```python
from build123d import *

# Parameters (mm, degrees)
BOSS_EXTRUDE1_DEPTH     = 3.7338
BOSS_EXTRUDE2_DEPTH     = 3.7338
CUT_EXTRUDE1_DEPTH      = 197.398400929
FILLET7_R               = 9.525
FILLET8_R               = 3.175
F_8_32_TAPPED_HOLE2_D   = 4.1656
FILLET3_RADIUS          = 1.8669
FILLET3_LENGTH          = 19.05
FILLET4_RADIUS          = 1.8669
FILLET4_LENGTH          = 19.05
FILLET5_RADIUS          = 1.8669
FILLET5_LENGTH          = 19.05
FILLET6_START           = -20
FILLET6_DEPTH           = 25
F_8_CLEARANCE_HOLE1_D   = 4.4958
CUT_EXTRUDE2_DEPTH      = 196.843388239
CUT_EXTRUDE3_DEPTH      = 196.843388239
SKETCH15_W              = 95.363977372
SKETCH15_H              = 7.9375
CUT_EXTRUDE4_DEPTH      = 196.843388239
SKETCH16_W              = 18.936022628
SKETCH16_H              = 6.35
CUT_EXTRUDE5_DEPTH      = 196.843388239
CUT_EXTRUDE6_DEPTH      = 196.843388239
CUT_EXTRUDE6_DEPTH_BACK = 196.843388239
SKETCH17_W              = 3.175
SKETCH17_H              = 3.175
SKETCH18_W              = 25.4
SKETCH18_H              = 3.175
CUT_EXTRUDE7_DEPTH      = 196.843388239


with BuildPart() as part:
    # Sketch1 → Boss-Extrude1 (new body)
    with BuildSketch(Plane.XY):
        Polygon((0, 0), (9.525, 0), (9.525, -19.05), (20.6375, -19.05), (20.6375, 0), (46.0375, 0), (46.0375, -19.05), (180.975, -19.05), (180.975, 3.175), (-16.893133293, 76.2), align=None)
    extrude(amount=BOSS_EXTRUDE1_DEPTH)

    # Sketch7 → Boss-Extrude2 (add)
    with BuildSketch(Plane.XY.offset(3.7338)):
        Polygon((-161.613635382, -74.129081959), (-0.247657199, 1.117109433), (-16.893133293, 76.2), (-166.605179671, -63.424680687), align=None)
    extrude(amount=-BOSS_EXTRUDE2_DEPTH)

    # Sketch8 → Cut-Extrude1 (cut, through all)
    with BuildSketch(Plane.XY.offset(3.7338)):
        Polygon((2.518832326, 10.642109433), (133.231722564, 10.642109433), (-9.128883742, 63.181561352), align=None)
        Polygon((-18.542737866, 61.637057548), (-138.674453357, -50.400369109), (-7.28718114, 10.86652211), align=None)
    extrude(amount=-CUT_EXTRUDE1_DEPTH, mode=Mode.SUBTRACT)

    # Fillet7
    fillet7_edges = [part.edges().sort_by_distance(p)[0] for p in [
        (-16.893133293, 76.2, 1.8669),
    ]]
    fillet(fillet7_edges, radius=FILLET7_R)

    # Fillet8
    fillet8_edges = [part.edges().sort_by_distance(p)[0] for p in [
        (-9.128883742, 63.181561352, 1.8669),
        (133.231722564, 10.642109433, 1.8669),
        (2.518832326, 10.642109433, 1.8669),
        (-7.28718114, 10.86652211, 1.8669),
        (-138.674453357, -50.400369109, 1.8669),
        (-18.542737866, 61.637057548, 1.8669),
    ]]
    fillet(fillet8_edges, radius=FILLET8_R)

    # #8-32 Tapped Hole2 (through all)
    with Locations(Plane.XY.offset(3.7338)):
        with Locations((15.08125, -11.1125), (58.7375, -11.1125), (168.275, -4.7625)):
            Hole(F_8_32_TAPPED_HOLE2_D / 2)

    # Fillet3: full round fillet: the end face becomes a half cylinder, R = half its width
    fillet3_face = Plane((9.525, -9.525, 1.8669), x_dir=(0, 1, 0), z_dir=(-1, 0, 0))  # on the end face: x along it, z out of the body
    fillet3_slab = fillet3_face.offset(-FILLET3_RADIUS / 2) * Box(FILLET3_LENGTH, 2 * FILLET3_RADIUS, FILLET3_RADIUS, mode=Mode.PRIVATE)  # the body's end, R deep
    fillet3_round = Plane((11.3919, -9.525, 1.8669), x_dir=(-1, 0, 0), z_dir=(0, 1, 0)) * Cylinder(FILLET3_RADIUS, FILLET3_LENGTH, mode=Mode.PRIVATE)  # its axis R under the face
    add(fillet3_slab - fillet3_round, mode=Mode.SUBTRACT)

    # Fillet4: full round fillet: the end face becomes a half cylinder, R = half its width
    fillet4_face = Plane((20.6375, -9.525, 1.8669), x_dir=(0, 1, 0), z_dir=(1, 0, 0))  # on the end face: x along it, z out of the body
    fillet4_slab = fillet4_face.offset(-FILLET4_RADIUS / 2) * Box(FILLET4_LENGTH, 2 * FILLET4_RADIUS, FILLET4_RADIUS, mode=Mode.PRIVATE)  # the body's end, R deep
    fillet4_round = Plane((18.7706, -9.525, 1.8669), x_dir=(1, 0, 0), z_dir=(0, 1, 0)) * Cylinder(FILLET4_RADIUS, FILLET4_LENGTH, mode=Mode.PRIVATE)  # its axis R under the face
    add(fillet4_slab - fillet4_round, mode=Mode.SUBTRACT)

    # Fillet5: full round fillet: the end face becomes a half cylinder, R = half its width
    fillet5_face = Plane((46.0375, -9.525, 1.8669), x_dir=(0, -1, 0), z_dir=(-1, 0, 0))  # on the end face: x along it, z out of the body
    fillet5_slab = fillet5_face.offset(-FILLET5_RADIUS / 2) * Box(FILLET5_LENGTH, 2 * FILLET5_RADIUS, FILLET5_RADIUS, mode=Mode.PRIVATE)  # the body's end, R deep
    fillet5_round = Plane((47.9044, -9.525, 1.8669), x_dir=(-1, 0, 0), z_dir=(0, -1, 0)) * Cylinder(FILLET5_RADIUS, FILLET5_LENGTH, mode=Mode.PRIVATE)  # its axis R under the face
    add(fillet5_slab - fillet5_round, mode=Mode.SUBTRACT)

    # Fillet6: read off the stored shape, not the designer's step
    # Fillet6 outline → Fillet6 (cut)
    with BuildSketch(Plane(origin=(0, 0, 0), x_dir=(1, 0, 0), z_dir=(0, 1, 0)).offset(FILLET6_START)):
        with BuildLine():
            ThreePointArc((179.1081, 0), (180.42819765, -0.54680235), (180.975, -1.8669))
            Line((180.975, -1.8669), (180.975, 0))
            Line((180.975, 0), (179.1081, 0))
        make_face()
        with BuildLine():
            ThreePointArc((180.975, -1.8669), (180.42819765, -3.18699765), (179.1081, -3.7338))
            Line((179.1081, -3.7338), (180.975, -3.7338))
            Line((180.975, -3.7338), (180.975, -1.8669))
        make_face()
    extrude(amount=FILLET6_DEPTH, mode=Mode.SUBTRACT)

    # #8 Clearance Hole1 (through all)
    with Locations(Plane.XY.offset(3.7338)):
        with Locations((-158.829891599, -65.073459713), (-124.299564913, -48.97170394)):
            Hole(F_8_CLEARANCE_HOLE1_D / 2)

    # Sketch12 → Cut-Extrude2 (cut, through all)
    with BuildSketch(Plane.XY.offset(3.7338)):
        Polygon((-0.247657199, 1.117109433), (0, 1.232593882), (0, 0), align=None)
    extrude(amount=-CUT_EXTRUDE2_DEPTH, mode=Mode.SUBTRACT)

    # Sketch14 → Cut-Extrude3 (cut, through all)
    with BuildSketch(Plane.XY.offset(3.7338)):
        with BuildLine():
            Line((71.4375, -6.35), (157.276477372, -6.35))
            ThreePointArc((157.276477372, -6.35), (162.038977372, -11.1125), (157.276477372, -15.875))
            Line((157.276477372, -15.875), (71.4375, -15.875))
            ThreePointArc((71.4375, -15.875), (66.675, -11.1125), (71.4375, -6.35))
        make_face()
    extrude(amount=-CUT_EXTRUDE3_DEPTH, mode=Mode.SUBTRACT)

    # Sketch15 → Cut-Extrude4 (cut, through all)
    with BuildSketch(Plane.XY.offset(3.7338)):
        with Locations((114.356988686, -15.08125)):
            Rectangle(SKETCH15_W, SKETCH15_H)
    extrude(amount=-CUT_EXTRUDE4_DEPTH, mode=Mode.SUBTRACT)

    # Sketch16 → Cut-Extrude5 (cut, through all)
    with BuildSketch(Plane.XY.offset(3.7338)):
        with Locations((171.506988686, -15.875)):
            Rectangle(SKETCH16_W, SKETCH16_H)
    extrude(amount=-CUT_EXTRUDE5_DEPTH, mode=Mode.SUBTRACT)

    # Sketch17 → Cut-Extrude6 (cut, two sides: drawn at the far end of the back side and taken through both)
    with BuildSketch(Plane.XY.offset(3.7338).offset(-CUT_EXTRUDE6_DEPTH_BACK)):
        with Locations((19.05, -17.4625)):
            Rectangle(SKETCH17_W, SKETCH17_H)
    extrude(amount=CUT_EXTRUDE6_DEPTH + CUT_EXTRUDE6_DEPTH_BACK, mode=Mode.SUBTRACT)

    # Sketch18 → Cut-Extrude7 (cut, through all)
    with BuildSketch(Plane.XY.offset(3.7338)):
        Polygon((-3.347186663, 3.175), (-2.005373682, 0.297472776), (0, 1.232593882), (0, 0), (9.525, 0), (9.525, 3.175), align=None)
        Polygon((-116.86007736, -49.756930231), (-115.518264379, -52.634457455), (-2.005373682, 0.297472776), (-3.347186663, 3.175), align=None)
        with Locations((33.3375, 1.5875)):
            Rectangle(SKETCH18_W, SKETCH18_H)
        with BuildLine():
            ThreePointArc((157.276477372, -6.35), (160.644073417, -7.744903955), (162.038977372, -11.1125))
            Line((162.038977372, -11.1125), (162.038977372, 3.175))
            Line((162.038977372, 3.175), (66.675, 3.175))
            Line((66.675, 3.175), (66.675, -11.1125))
            ThreePointArc((66.675, -11.1125), (68.069903955, -7.744903955), (71.4375, -6.35))
            Line((71.4375, -6.35), (157.276477372, -6.35))
        make_face()
    extrude(amount=-CUT_EXTRUDE7_DEPTH, mode=Mode.SUBTRACT)


solid = part.part
```
For this review, take the finished solid that the model builds, in its own axes (mm). A direction names the side the tool comes from. Coordinates: 2 decimals unless noted, no trailing zeros. Loops run counter-clockwise (first coordinate to the right, second up) from the corner with the lowest first, then second, coordinate; pieces in that order, holes last. Notation, with made-up numbers: (33.5, 51) - (68.5, 51) arc R15 cw to (68.5, 57) - close; hole circle Ø5 at (43, 28.5). An arc over 180 degrees is marked (long way). Use one line per item in the form item = value. Start each with the question number.
1) Take a section at D-D (z = 2.8). State how many separate pieces and enclosed holes the cut face has, plus the area to 3 significant figures.
2) Take a section at A-A (x = -50.5). State the section outline as (y, z) points, plus the area to 3 significant figures.
3) Take a section at C-C (x = 103.5). State the section outline as (y, z) points (3 decimals).
4) Draft analysis for pull direction Y (two halves, no side actions). For faces 1 (the face through (-72.6, 11.22, 1.89)), 2 (the face through (-92.876, 5.336, 1.893)), 3 (the face through (-7, 6, 0)), state which applies: released by +Y, released by -Y, zero draft, split by the parting line, or undercut.
5) Take a section at B-B (y = 26). State the section outline as (x, z) points, plus the area to 3 significant figures.
6) For pin 1 (1.1 mm diameter, centred on x = 57.5, z = 1.5, fed in from -Y); pin 2 (2 mm diameter, centred on x = -34, z = 3, fed in from -Y); pin 3 (0.9 mm diameter, centred on x = 19.5, z = 0.5, fed in from -Y) (3 decimals), all flat-tipped, find the tip position at first contact; note any pin that passes through.
7) For faces 4 (the face through (-3.02, 35.63, 1.89)), 5 (the face through (86.139, 38.175, 1.841)), list the 3-axis set-ups (+Z, -Z, +X, -X, +Y, -Y) from which the entire face can be reached by the end or side of a thin tool; tool diameter is ignored.
8) To check wall thickness, follow probe 1 along X at (y, z) = (-8.5, 1.45) (3 decimals); probe 2 along Y at (x, z) = (-29, 3.15); probe 3 along Y at (x, z) = (-88, 0.7). State the ranges of each line that lie inside material, in increasing order. Write a range as from..to.
From the geometry:
q1.separate_pieces = 1
q1.enclosed_holes = 7
q1.area = 7,960 mm2
q2.outline = (-18.81, 0) - (-9.28, 0) - (-9.28, 3.73) - (-18.81, 3.73) - close; (31.83, 0) - (44.86, 0) - (44.86, 3.73) - (31.83, 3.73) - close
q2.area = 84.2 mm2
q3.outline = (3.175, 0) - (10.642, 0) - (10.642, 3.734) - (3.175, 3.734) - close; (21.615, 0) - (31.768, 0) - (31.768, 3.734) - (21.615, 3.734) - close
q4.face_1 = undercut
q4.face_2 = released by +Y
q4.face_3 = zero draft
q5.outline = (-70.72, 0) - (-56.75, 0) - (-56.75, 3.73) - (-70.72, 3.73) - close; (-10.64, 0) - (-0.89, 0) - (-0.89, 3.73) - (-10.64, 3.73) - close; (91.62, 0) - (119.13, 0) - (119.13, 3.73) - (91.62, 3.73) - close
q5.area = 191 mm2
q6.pin_1 = -19.05
q6.pin_2 = -11.58
q6.pin_3 = -15.875
q7.face_4 = +Z, -Z
q7.face_5 = +Z, -Z, +X, +Y
q8.probe_1 = -107.712..-93.747, -48.819..-28.384, 9.572..20.59, 46.085..66.675, 162.039..180.928
q8.probe_2 = -8.79..0.74, 51.88..64.91
q8.probe_3 = -36.3..-26.77, -3.14..9.88
